Part model, mm, in its own coordinate system. A direction names the side the tool comes from. Coordinates: 2 decimals unless noted, no trailing zeros. Loops run counter-clockwise (first coordinate to the right, second up) from the corner with the lowest first, then second, coordinate; pieces in that order, holes last. Notation, with made-up numbers: (28.25, -29.75) - (87.25, -29.75) arc R26 ccw to (87.25, -8.75) - close; hole circle Ø8 at (-33.75, 23). An arc over 180 degrees is marked (long way). Use a Markdown table: item, result. Add a question column.
1) Drop flat-ended pins along their axis: P1, Ø3, axis at y = 107.5, z = 286.5, coming from the -X side; P2, Ø7.5, axis at x = 533, y = -97, coming from the +Z side; P3, Ø2, axis at y = -269, z = 290.5, coming from the -X side. Give the stop position or say it passes through.
2) Probe probe 1 along X at (y, z) = (-295.5, 415); probe 2 along Z at (x, y) = (901, -298.5); probe 3 along X at (y, z) = (213, 312). List the from-to ranges inside material, lowest first. Write a range as [from, to].
3) Band-saw the part on A-A (y = 91). Give the cut face in (x, z), plus the area to 3 significant figures.
4) Band-saw the part on B-B (z = 254). Give the cut face in (x, y).
5) Tool access for faces 1 (the face through (639.391, -266.398, 187.934)), 2 (the face through (531, -3, 106.791)): list every direction of +Z, -Z, +X, -X, +Y, -Y with a clear straight run to the whole face (end or side of a thin tool).
6) Band-saw the part on C-C (x = 834.5). Give the cut face in (y, z).
from build123d import *

# Parameters (mm, degrees)
WYCI_GNI_CIE_CIENKA_CIANKA1_DEPTH      = 400
WYCI_GNI_CIE_CIENKA_CIANKA1_DEPTH_BACK = 400
LUSTRO1_START                          = 275.975094607
LUSTRO1_DEPTH                          = 4


# Read off the part's stored shape, not the designer's step: Lustro1
with BuildPart() as part:
    # Szkic1 → Wyciągnięcie-cienka ścianka1 (new, two sides: drawn at the far end of the back side and taken through both)
    with BuildSketch(Plane(origin=(0, 0, 0), x_dir=(1, 0, 0), z_dir=(0, 1, 0)).offset(-WYCI_GNI_CIE_CIENKA_CIANKA1_DEPTH_BACK)):
        Polygon((958.263871938, -462.035437036), (545, -102.790633942), (517.881642578, -102.790633942), (517.881642578, -106.790633942), (543.504461282, -106.790633942), (955.639635822, -465.054275357), align=None)
    extrude(amount=WYCI_GNI_CIE_CIENKA_CIANKA1_DEPTH + WYCI_GNI_CIE_CIENKA_CIANKA1_DEPTH_BACK)

    # Cięcie powierzchnią3
    split(bisect_by=Plane(origin=(-14.708403282, 64.029657214, -16.335336758), x_dir=(0.6328754019355285, 0.32469887066665293, 0.7028793417171568), z_dir=(0.2172659522131463, -0.9458174471787886, 0.2412982855743377)), keep=Keep.TOP)

    # Cięcie powierzchnią4
    split(bisect_by=Plane(origin=(-14.708403282, -64.029657214, -16.335336758), x_dir=(0.6328754019353329, -0.32469887066665304, 0.7028793417173329), z_dir=(-0.21726595221314635, -0.9458174471787884, -0.24129828557433775)), keep=Keep.BOTTOM)

    # Cięcie powierzchnią5
    split(bisect_by=Plane(origin=(141.124135037, -578.697205105, 122.677338974), x_dir=(0.718149384400474, 0.30747157670526803, 0.6242777356302215), z_dir=(0.2320517445856664, -0.9515572654960797, 0.20171950405543876)), keep=Keep.BOTTOM)

    # Cięcie powierzchnią6
    split(bisect_by=Plane(origin=(-23.206221207, -200.985361995, -20.17286033), x_dir=(0.74602943431762, -0.15122940248105377, 0.6485134932728503), z_dir=(-0.11413427886381658, -0.9884986938915112, -0.09921541494653495)), keep=Keep.BOTTOM)

    # Lustro1 outline → Lustro1 (cut)
    with BuildSketch(Plane(origin=(0, 0, 0), x_dir=(0.754709580222771, 0, 0.6560590289905084), z_dir=(0.6560590289905085, 0, -0.7547095802227708)).offset(LUSTRO1_START)):
        Polygon((1026.333444714, -307.485100364), (910.348198503, -344.962788591), (775.810550903, -324.380011716), (774, -324.103017388), (774, -400), (1026.333444714, -400), align=None)
    extrude(amount=LUSTRO1_DEPTH, mode=Mode.SUBTRACT)


solid = part.part
Answer block:
| question | item | result |
|---|---|---|
| 1 | P1 | x = 748.51 |
| 1 | P2 | z = 106.79 |
| 1 | P3 | x = 753.69 |
| 2 | probe 1 | [898.06, 904.16] |
| 2 | probe 2 | [412.26, 417.56] |
| 2 | probe 3 | [779.57, 785.67] |
| 3 | outline | (517.88, 102.79) - (545, 102.79) - (958.26, 462.04) - (955.64, 465.05) - (543.5, 106.79) - (517.88, 106.79) - close |
| 3 | area | 2,290 mm2 |
| 4 | outline | (712.85, -300.13) - (718.95, -301.53) - (718.95, 301.53) - (712.85, 300.13) - close |
| 5 | face 1 | -Z, -X, -Y |
| 5 | face 2 | +Z, -X, +Y, -Y |
| 6 | outline | (-338.15, 359.75) - (-337.62, 354.45) - (337.62, 354.45) - (338.15, 359.75) - close |
